from build123d import *

# Parameters (mm, degrees)
BOSS_EXTRUDE1_DEPTH  = 30
SKETCH2_W            = 30
SKETCH2_H            = 300
BOSS_EXTRUDE2_DEPTH  = 30
SKETCH3_W            = 30
SKETCH3_H            = 30
BOSS_EXTRUDE3_DEPTH  = 800
SKETCH4_W            = 1200
SKETCH4_H            = 30
BOSS_EXTRUDE4_DEPTH  = 30
BOSS_EXTRUDE5_REACH  = 1367.394
SKETCH5_W            = 1100
SKETCH5_H            = 30
BOSS_EXTRUDE6_REACH  = 1350.814
SKETCH6_W            = 30
SKETCH6_H            = 30
SKETCH7_R            = 20
BOSS_EXTRUDE9_DEPTH  = 240
BOSS_EXTRUDE10_START = -240
BOSS_EXTRUDE10_DEPTH = 240
SKETCH9_R            = 6
CUT_EXTRUDE1_DEPTH   = 100


with BuildPart() as part:
    # Sketch1 → Boss-Extrude1 (new body)
    with BuildSketch(Plane.XY):
        Polygon((0, 0), (0, 800), (-150, 800), (-150, 830), (1050, 830), (1050, 800), (900, 800), (900, 0), (870, 0), (870, 800), (30, 800), (30, 0), align=None)
    extrude(amount=BOSS_EXTRUDE1_DEPTH)

    # Sketch2 → Boss-Extrude2 (add)
    with BuildSketch(Plane.XZ):
        with Locations((15, 150)):
            Rectangle(SKETCH2_W, SKETCH2_H)
        with Locations((885, 150)):
            Rectangle(SKETCH2_W, SKETCH2_H)
    extrude(amount=BOSS_EXTRUDE2_DEPTH)

    # Sketch3 → Boss-Extrude3 (add)
    with BuildSketch(Plane(origin=(0, 0, 0), x_dir=(1, 0, 0), z_dir=(0, 1, 0))):
        with Locations((15, -285)):
            Rectangle(SKETCH3_W, SKETCH3_H)
        with Locations((885, -285)):
            Rectangle(SKETCH3_W, SKETCH3_H)
    extrude(amount=BOSS_EXTRUDE3_DEPTH)

    # Sketch4 → Boss-Extrude4 (add)
    with BuildSketch(Plane(origin=(0, 800, 0), x_dir=(1, 0, 0), z_dir=(0, 1, 0))):
        with Locations((450, -285)):
            Rectangle(SKETCH4_W, SKETCH4_H)
    extrude(amount=BOSS_EXTRUDE4_DEPTH)

    # Sketch5 → Boss-Extrude5 (add, up to next)
    with BuildSketch(Plane.XY.offset(30), mode=Mode.PRIVATE) as boss_extrude5_sk1:
        with Locations((450, 815)):
            Rectangle(SKETCH5_W, SKETCH5_H)
    boss_extrude5_tool1 = extrude(boss_extrude5_sk1.sketch, amount=BOSS_EXTRUDE5_REACH, mode=Mode.PRIVATE) - part.part
    add(boss_extrude5_tool1.solids().sort_by_distance((450, 815, 30))[0])

    # Sketch6 → Boss-Extrude6 (add, up to next)
    with BuildSketch(Plane(origin=(30, 0, 0), x_dir=(0, 0, -1), z_dir=(1, 0, 0)), mode=Mode.PRIVATE) as boss_extrude6_sk1:
        with Locations((-150, -15)):
            Rectangle(SKETCH6_W, SKETCH6_H)
    boss_extrude6_tool1 = extrude(boss_extrude6_sk1.sketch, amount=BOSS_EXTRUDE6_REACH, mode=Mode.PRIVATE) - part.part
    add(boss_extrude6_tool1.solids().sort_by_distance((30, -15, 150))[0])

    # Sketch7 → Boss-Extrude9 (add)
    with BuildSketch(Plane(origin=(0, 0, 270), x_dir=(-1, 0, 0), z_dir=(0, 0, -1))):
        with Locations(Location((-1025, 815, 0), (0, 0, 228.590377891))):
            Circle(SKETCH7_R)
        with Locations(Location((125, 815, 0), (0, 0, 228.590377891))):
            Circle(SKETCH7_R)
    extrude(amount=BOSS_EXTRUDE9_DEPTH)

    # Sketch8 → Boss-Extrude10 (add)
    with BuildSketch(Plane(origin=(0, 0, 30), x_dir=(-1, 0, 0), z_dir=(0, 0, -1)).offset(BOSS_EXTRUDE10_START)):
        with BuildLine():
            Line((125, 837), (-1025, 837))
            ThreePointArc((-1025, 837), (-1047, 815), (-1025, 793))
            Line((-1025, 793), (125, 793))
            ThreePointArc((125, 793), (147, 815), (125, 837))
        make_face()
        with BuildLine():
            Line((125, 835), (-1025, 835))
            ThreePointArc((-1025, 835), (-1045, 815), (-1025, 795))
            Line((-1025, 795), (125, 795))
            ThreePointArc((125, 795), (145, 815), (125, 835))
        make_face(mode=Mode.SUBTRACT)
    extrude(amount=BOSS_EXTRUDE10_DEPTH)

    # Sketch9 → Cut-Extrude1 (cut)
    with BuildSketch(Plane.XZ.offset(30)):
        with Locations((15, 280)):
            Circle(SKETCH9_R)
        with Locations(Location((15, 20, 0), (0, 0, 180))):
            Circle(SKETCH9_R)
        with Locations((885, 20)):
            Circle(SKETCH9_R)
        with Locations(Location((885, 280, 0), (0, 0, 180))):
            Circle(SKETCH9_R)
    extrude(amount=-CUT_EXTRUDE1_DEPTH, mode=Mode.SUBTRACT)


solid = part.part
Geometry: final body of the model. Coordinates: model frame, mm. A direction names the side the tool comes from. Give positions to 0.01 mm unless a question says otherwise; leave off trailing zeros. Loops run counter-clockwise (first coordinate to the right, second up) from the corner with the lowest first, then second, coordinate; pieces in that order, holes last. Notation, with made-up numbers: M 15.5,51.25 L 44.5,51.25 A15 ccw 44.5,67.25 Z; hole C 2.5,83.25 d8. An arc over 180 degrees is marked long. Put each result on its own line as item: value.
1) Material intervals for L1, parallel to Y at x = 820, z = 208; L2, parallel to X at y = 33, z = 280; L3, parallel to Z at x = 885, y = 20.5, sorted ascending. Write a range as from..to.
Computed values:
L1: y = 793..795, 800..830, 835..837
L2: x = 0..9, 21..30, 870..879, 891..900
L3: z = 0..14, 26..30, 270..274, 286..300
2) Cut plane C-C, the plane y = 768. Return the cut outline in (x, z).
Computed values:
outline: M 0,0 L 30,0 L 30,30 L 0,30 Z; M 0,270 L 30,270 L 30,300 L 0,300 Z; M 870,0 L 900,0 L 900,30 L 870,30 Z; M 870,270 L 900,270 L 900,300 L 870,300 Z
3) First-contact query: P1, Ø8, axis at x = 89.5, z = 176, coming from the -Y side; P2, Ø11, axis at x = 15, z = 20, coming from the -Y side; P3, Ø1, axis at x = 614, y = 793.5, coming from the +Z side; P4, Ø3.5, axis at x = 992.5, y = 797, coming from the +Z side. Flat tips, straight axial feed; report the tip coordinate or a pass-through.
Computed values:
P1: stops at y = 793
P2: stops at y = 70
P3: stops at z = 270
P4: passes through
4) Cut plane B-B, the plane x = -70. Return the cut outline in (y, z), plus the area to 3 significant figures.
Computed values:
outline: M 793,30 L 795,30 L 795,270 L 793,270 Z; M 800,0 L 830,0 L 830,300 L 800,300 Z; M 835,30 L 837,30 L 837,270 L 835,270 Z
area: 9,960 mm^2
5) Cut plane A-A, the plane z = 249.5. Return the cut outline in (x, y), plus the area to 3 significant figures.
Computed values:
outline: M -125,793 L 1025,793 A22 ccw 1025,837 L -125,837 A22 ccw Z; M -100,800 L 1000,800 L 1000,830 L -100,830 Z; M 0,-30 L 30,-30 L 30,0 L 0,0 Z; M 870,-30 L 900,-30 L 900,0 L 870,0 Z; hole M -125,795 L 1025,795 A20 cw 1025,835 L -125,835 A20 cw Z
area: 42,200 mm^2
6) Cut plane D-D, the plane x = 536. Return the cut outline in (y, z).
Computed values:
outline: M -30,135 L 0,135 L 0,165 L -30,165 Z; M 793,30 L 795,30 L 795,270 L 793,270 Z; M 800,0 L 830,0 L 830,300 L 800,300 Z; M 835,30 L 837,30 L 837,270 L 835,270 Z
7) Mould query, pull axis X, two halves, no side actions, for faces 1 (the flat face through (442, 837, 152)), 2 (the flat face through (-150, 815, 285)), 3 (the flat face through (-100, 815, 148)), 4 (the flat face through (444, -15, 165)). Classes: released by +X, released by -X, zero draft, split by the parting line, or undercut.
Computed values:
face 1: zero draft
face 2: released by -X
face 3: undercut
face 4: undercut
8) Reachability of faces 5 (the flat face through (442, 835, 152)), 6 (the cylindrical face through (1047, 815, 152)), 7 (the flat face through (885, 402, 30)), 8 (the flat face through (30, 322, 23)) from +Z, -Z, +X, -X, +Y, -Y: full face, straight path, thin tool, end or side. Return the list, or none.
Computed values:
face 5: +Z, -Z
face 6: +X
face 7: +X, -X
face 8: -Z, -Y
